Read the model definition and answer for the solid it produces. Units are mm, in the model's axes. Face numbers are marked on the shaded views. A direction names the side the tool comes from. Round coordinates to 2 decimals unless told otherwise and drop trailing zeros. Loops run counter-clockwise (first coordinate to the right, second up) from the corner with the lowest first, then second, coordinate; pieces in that order, holes last. Notation, with made-up numbers: (46.5, 40.25) - (75.5, 40.25) arc R20 cw to (75.5, 78.25) - close; hole circle Ø6 at (-12.75, 58.25). An arc over 180 degrees is marked (long way). Use CSV: the item, a comma, the result in double quotes. Start each with the question number.
1. Find section C-C (y = -9). Give the vertices of the cut face in (x, z).
2. Consider line 1 along Z through (x, y) = (-0.5, -3); line 2 along X through (y, z) = (-11, 7.5); line 3 along X through (y, z) = (-33, 4). Determine where each line is inside the solid, lowest interval first.
3. Given pin 1 Ø4 at (x, y) = (1, -36) entering from -Z; pin 2 Ø1.5 at (x, z) = (-11, 3) entering from -Y; pin 3 Ø12 at (y, z) = (-17.5, -7) entering from +X; pin 4 Ø3 at (x, y) = (-11.5, -32.5) entering from +Z, each flat-ended and moving along its own axis, determine where each tip first touches the part or whether it passes through.
4. Find section B-B (x = 0). Give the vertices of the cut face in (y, z), and give its area (3 significant figures).
5. A tool of negligible diameter and unlimited length cuts with its end or side. For the marked faces 1 and 2, from which of +Z, -Z, +X, -X, +Y, -Y can it reach the whole face along a straight path? Write none if from no direction.
6. Find section D-D (y = -21.5). Give the vertices of the cut face in (x, z), and give its area (3 significant figures).
7. Find section A-A (z = 0). Give the vertices of the cut face in (x, y), and give its area (3 significant figures).
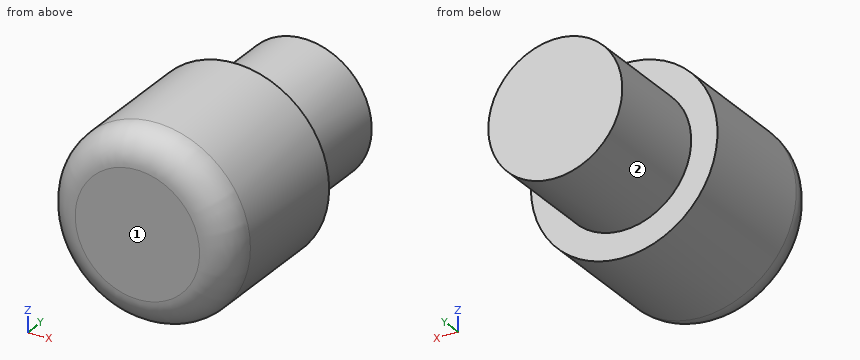
from build123d import *

# Parameters (mm, degrees)
F0_R     = 10.9474
F1_DEPTH = 17.78
F2_R     = 15.24
F2_R_2   = 10.9474
F3_DEPTH = 25.4
F4_R     = 5.08


with BuildPart() as f1:
    # F0 (on Front) → F1 (new body)
    with BuildSketch(Plane.XZ):
        Circle(F0_R)
    extrude(amount=F1_DEPTH)

    # F2 (on face) → F3 (join)
    with BuildSketch(Plane.XZ.offset(17.78)):
        Circle(F2_R)
        Circle(F2_R_2, mode=Mode.SUBTRACT)
        Circle(F2_R_2)
    extrude(amount=F3_DEPTH)

    # F4
    f4_edges = [f1.edges().sort_by_distance(p)[0] for p in [
        (-15.24, -43.18, 0),
    ]]
    fillet(f4_edges, radius=F4_R)


solid = f1.part
Filled sheet:
1,outline,"circle Ø21.89 at (0, 0)"
2,line 1,"z = -10.94 to 10.94"
2,line 2,"x = -7.97 to 7.97"
2,line 3,"x = -14.71 to 14.71"
3,pin 1,"stops at z = -15.24"
3,pin 2,"stops at y = -43.16"
3,pin 3,"stops at x = 15.21"
3,pin 4,"stops at z = 11.5"
4,outline,"(-43.18, -10.16) arc R5.08 ccw to (-38.1, -15.24) - (-17.78, -15.24) - (-17.78, -10.95) - (0, -10.95) - (0, 10.95) - (-17.78, 10.95) - (-17.78, 15.24) - (-38.1, 15.24) arc R5.08 ccw to (-43.18, 10.16) - close"
4,area,"1,150 mm²"
5,face 1,"+Z, -Z, +X, -X, -Y"
5,face 2,"+Y"
6,outline,"circle Ø30.48 at (0, 0)"
6,area,"730 mm²"
7,outline,"(-15.24, -38.1) arc R5.08 ccw to (-10.16, -43.18) - (10.16, -43.18) arc R5.08 ccw to (15.24, -38.1) - (15.24, -17.78) - (10.95, -17.78) - (10.95, 0) - (-10.95, 0) - (-10.95, -17.78) - (-15.24, -17.78) - close"
7,area,"1,150 mm²"
